```python
from build123d import *

# Parameters (mm, degrees)
SKETCH1_R           = 4
BOSS_EXTRUDE1_DEPTH = 6.35
FILLET1_R           = 2
FILLET2_R           = 3


with BuildPart() as part:
    # Sketch1 → Boss-Extrude1 (new body)
    with BuildSketch(Plane(origin=(0, 0, 0), x_dir=(1, 0, 0), z_dir=(0, 1, 0))):
        with BuildLine():
            Line((0, -12.5), (50, -12.5))
            Line((50, -12.5), (50, -6.5))
            Line((50, -6.5), (0, 12.5))
            ThreePointArc((0, 12.5), (-12.5, 0), (0, -12.5))
        make_face()
        with Locations(Location((0, 0, 0), (0, 0, 270))):
            Circle(SKETCH1_R, mode=Mode.SUBTRACT)
    extrude(amount=BOSS_EXTRUDE1_DEPTH)

    # Fillet1
    fillet1_edges = [part.edges().sort_by_distance(p)[0] for p in [
        (50, 3.175, 6.5),
        (50, 3.175, 12.5),
    ]]
    fillet(fillet1_edges, radius=FILLET1_R)

    # Fillet2
    fillet2_edges = [part.edges().sort_by_distance(p)[0] for p in [
        (0, 3.175, -12.5),
    ]]
    fillet(fillet2_edges, radius=FILLET2_R)


solid = part.part
```
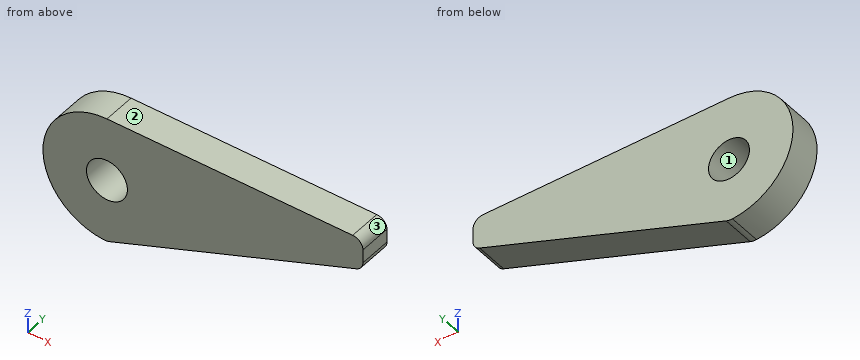
Model file for the job. Use its own axes, mm. Face numbers are marked on the shaded views. Coordinates: 2 decimals unless noted, no trailing zeros. Order: outer loops, then holes, each group sorted by start corner. A loop starts at its lowest first (then second) coordinate and runs counter-clockwise, first axis right, second up. Notation, with made-up numbers: M 68,28.5 L 74,28.5 A31 cw 74,59.5 Z; hole C 46,34 d8. An arc over 180 degrees is marked long. Answer as CSV lines item,"result".
(1) Band-saw the part on B-B, the plane z = 1. List the corners of the cut face in (x, y), then the cut area to 3 significant figures.
Geometry says:
outline,"M -12.46,0 L -3.87,0 L -3.87,6.35 L -12.46,6.35 Z; M 3.87,0 L 35.53,0 L 35.53,6.35 L 3.87,6.35 Z"
area,"256 mm2"
(2) Band-saw the part on A-A, the plane y = 2. List the corners of the cut face in (x, z).
Geometry says:
outline,"M -0.68,-12.48 A3 ccw 0.55,-12.29 L 48.71,6.01 A2 ccw 50,7.88 L 50,10.5 A2 ccw 48,12.5 L 0,12.5 A12.5 ccw Z; hole C 0,0 d8"
(3) Band-saw the part on C-C, the plane x = 39. List the corners of the cut face in (y, z).
Geometry says:
outline,"M 0,2.32 L 6.35,2.32 L 6.35,12.5 L 0,12.5 Z"
(4) Pull direction X, two halves, no side cores. Call the marked faces 1, 2 and 3: +X half, -X half, draft (parallel to the pull), parting line (faces both ways), or undercut.
Geometry says:
face 1,"undercut"
face 2,"draft"
face 3,"+X half"
(5) Flat gauge pin, fed straight in: pin 1 (1 mm diameter, centred on x = 0, y = 5, fed in from -Z). Where does the tip first touch, or does it go through?
Geometry says:
pin 1,"stops at z = -12.49"
(6) Band-saw the part on D-D, the plane z = -4.75. List the corners of the cut face in (x, y), then the cut area to 3 significant figures.
Geometry says:
outline,"M -11.56,0 L 20.39,0 L 20.39,6.35 L -11.56,6.35 Z"
area,"203 mm2"
(7) Wall check: line 1 along Z through (x, y) = (-2.5, 6); line 2 along Z through (x, y) = (16, 3.25); line 3 along Z through (x, y) = (11, 2.75). Give the ranges that are in metal, low to high.
Geometry says:
line 1,"z = -12.25 to -3.12, 3.12 to 12.25"
line 2,"z = -6.42 to 12.5"
line 3,"z = -8.32 to 12.5"
